from build123d import *

# Parameters (mm, degrees)
F1_DEPTH  = 25.4
F2_R      = 1.5875
F3_DEPTH  = 49.022
F4_R      = 3.96875
F5_DEPTH  = 25.4
F6_R      = 1.4097
F7_DEPTH  = 25.4
F9_R      = 2.3876
F10_DEPTH = 3.175
F11_R     = 0.99695
F12_DEPTH = 12.7
F13_R     = 1.5875
F14_DEPTH = 13.716


with BuildPart() as f1:
    # F0 (on Front) → F1 (new body)
    with BuildSketch(Plane.XZ):
        Polygon((0, 25.4), (0, 0), (25.4, 0), (25.4, 60.325), (12.7, 60.325), (12.7, 25.4), align=None)
    extrude(amount=F1_DEPTH)

    # F2 (on face) → F3 (cut)
    with BuildSketch(Plane.XY.offset(60.325)):
        with Locations((19.05, -12.7)):
            Circle(F2_R)
    extrude(amount=-F3_DEPTH, mode=Mode.SUBTRACT)

    # F4 (on face) → F5 (cut)
    with BuildSketch(Plane(origin=(0, 0, 0), x_dir=(0, -1, 0), z_dir=(-1, 0, 0))):
        with Locations((12.7, 12.7)):
            Circle(F4_R)
    extrude(amount=-F5_DEPTH, mode=Mode.SUBTRACT)

    # F6 (on face) → F7 (cut)
    with BuildSketch(Plane(origin=(12.7, 0, 0), x_dir=(0, -1, 0), z_dir=(-1, 0, 0))):
        with Locations((4.7752, 53.975)):
            Circle(F6_R)
        with Locations((4.7752, 41.275)):
            Circle(F6_R)
        with Locations((20.6248, 53.975)):
            Circle(F6_R)
        with Locations((20.6248, 41.275)):
            Circle(F6_R)
    extrude(amount=-F7_DEPTH, mode=Mode.SUBTRACT)

    # F9 (on face) → F10 (cut)
    with BuildSketch(Plane(origin=(12.7, 0, 0), x_dir=(0, -1, 0), z_dir=(-1, 0, 0))):
        with Locations((4.7752, 53.975)):
            Circle(F9_R)
        with Locations((4.7752, 41.275)):
            Circle(F9_R)
        with Locations((20.6248, 41.275)):
            Circle(F9_R)
        with Locations((20.6248, 53.975)):
            Circle(F9_R)
    extrude(amount=-F10_DEPTH, mode=Mode.SUBTRACT)

    # F11 (on face) → F12 (cut)
    with BuildSketch(Plane(origin=(0, 0, 0), x_dir=(1, 0, 0), z_dir=(0, 0, -1))):
        with Locations((12.7, 19.05)):
            Circle(F11_R)
        with Locations((12.7, 6.35)):
            Circle(F11_R)
    extrude(amount=-F12_DEPTH, mode=Mode.SUBTRACT)

    # F13 (on face) → F14 (cut)
    with BuildSketch(Plane.XY.offset(25.4)):
        with Locations((6.35, -12.7)):
            Circle(F13_R)
    extrude(amount=-F14_DEPTH, mode=Mode.SUBTRACT)


solid = f1.part
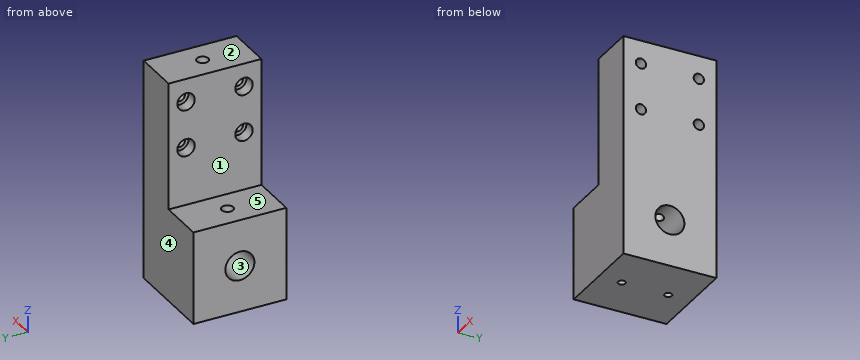
Model file for the job. Use its own axes, mm. Face numbers are marked on the shaded views. A direction names the side the tool comes from. Give positions to 0.01 mm unless a question says otherwise; leave off trailing zeros. Order: outer loops, then holes, each group sorted by start corner. A loop starts at its lowest first (then second) coordinate and runs counter-clockwise, first axis right, second up. Notation, with made-up numbers: M -30.5,20 L 5.5,20 A37 ccw 5.5,57 Z; hole C 3,57 d1. An arc over 180 degrees is marked long. Write item = value, one per line.
Q1. Cut at D-D, the plane z = 17.5. Count the separate pieces of the cut face and the enclosed holes in it, then the cut area to 3 significant figures.
Derived:
separate_pieces = 1
enclosed_holes = 2
area = 629 mm2
Q2. Cut at A-A, the plane y = -12.7. List the corners of the cut face in (x, z) (1 decimal).
Derived:
outline = M 0,0 L 25.4,0 L 25.4,8.7 L 0,8.7 Z; M 0,16.7 L 4.8,16.7 L 4.8,25.4 L 0,25.4 Z; M 7.9,16.7 L 17.5,16.7 L 17.5,60.3 L 12.7,60.3 L 12.7,25.4 L 7.9,25.4 Z; M 20.6,16.7 L 25.4,16.7 L 25.4,60.3 L 20.6,60.3 Z
Q3. Drill centre lines: line 1 (X direction, y = -12.7, z = 30); line 2 (Y direction, x = 19.25, z = 34); line 3 (Z direction, x = 11.5, y = -13.25). Where is each one in solid material? Low to high. Write a range as [from, to].
Derived:
line_1 = [12.7, 17.46], [20.64, 25.4]
line_2 = [-25.4, -14.27], [-11.13, 0]
line_3 = [0, 8.77], [16.63, 25.4]
Q4. Flat gauge pins, fed straight in: pin 1 (10 mm diameter, centred on x = 6.5, z = 30, fed in from +Y); pin 2 (5.5 mm diameter, centred on y = -21.5, z = 40, fed in from -X); pin 3 (3 mm diameter, centred on y = -4.78, z = 53.98, fed in from -X) (3 decimals); pin 4 (2.5 mm diameter, centred on y = -4.78, z = 41.28, fed in from -X). Where does each tip first touch, or does it go through?
Derived:
pin_1 = 0
pin_2 = 12.7
pin_3 = 15.875
pin_4 = through
Q5. Cut at C-C, the plane x = 19.05. List the corners of the cut face in (y, z) (1 decimal), then the cut area to 3 significant figures.
Derived:
outline = M -25.4,0 L 0,0 L 0,60.3 L -11.1,60.3 L -11.1,16.3 A4 cw long -14.3,16.3 L -14.3,60.3 L -25.4,60.3 Z; hole C -20.6,41.3 d2.8; hole C -20.6,54 d2.8; hole C -4.8,41.3 d2.8; hole C -4.8,54 d2.8
area = 1,320 mm2
Q6. Tool access for the marked faces 4 and 5: list every direction of +Z, -Z, +X, -X, +Y, -Y with a clear straight run to the whole face (end or side of a thin tool).
Derived:
face_4 = +Z, -Z, +X, -X, +Y
face_5 = +Z, -X, +Y, -Y
Q7. Two-plate mould, pull along Z, no slides. Class the marked faces 1, 2 and 3: pulls with the +Z half, pulls with the -Z half, needs draft (parallel to the pull), parting line crosses it, or undercut.
Derived:
face_1 = needs draft
face_2 = pulls with the +Z half
face_3 = undercut
